from build123d import *

# Parameters (mm, degrees)
SKETCH1_R                  = 3.3782
BASE_FLANGE1_DEPTH         = 3.175
SKETCHED_START             = -12.7
SKETCHED_BEND1_DEPTH       = 25.4
SKETCHED_START_2           = -10.229596
SKETCHED_BEND1_2_DEPTH     = 6.8513959
SKETCHED_START_3           = 3.3782001
SKETCHED_BEND1_3_DEPTH     = 6.7817999
SKETCHED_BEND1_4_DEPTH     = 25.4
SKETCHED_START_4           = 9.775295033
SKETCHED_BEND1_5_OUTLINE_R = 3.3782
SKETCHED_BEND1_5_DEPTH     = 3.175


with BuildPart() as part:
    # Base-Flange1: sheet metal written as solids
    # Sketch1 → Base-Flange1 (new body)
    with BuildSketch(Plane.XY):
        with BuildLine():
            Line((-10.16, -25.4), (10.16, -25.4))
            ThreePointArc((10.16, -25.4), (11.956051224, -24.656051224), (12.7, -22.86))
            Line((12.7, -22.86), (12.7, 46.99))
            ThreePointArc((12.7, 46.99), (11.956051224, 48.786051224), (10.16, 49.53))
            Line((10.16, 49.53), (-10.16, 49.53))
            ThreePointArc((-10.16, 49.53), (-11.956051224, 48.786051224), (-12.7, 46.99))
            Line((-12.7, 46.99), (-12.7, -22.86))
            ThreePointArc((-12.7, -22.86), (-11.956051224, -24.656051224), (-10.16, -25.4))
        make_face()
        with Locations((0, 36.83)):
            Circle(SKETCH1_R, mode=Mode.SUBTRACT)
        with Locations((0, -12.7)):
            Circle(SKETCH1_R, mode=Mode.SUBTRACT)
    extrude(amount=-BASE_FLANGE1_DEPTH)

    # Sketched Bend1: read off the stored shape, not the designer's step
    # Sketched Bend1 outline → Sketched Bend1 (cut)
    with BuildSketch(Plane.YZ.offset(SKETCHED_START)):
        with BuildLine():
            Line((49.53, 0), (14.953712647, 0))
            Line((14.953712647, 0), (14.325844229, -1.0875))
            ThreePointArc((14.325844229, -1.0875), (12.797688168, -2.615656061), (10.710188168, -3.175))
            Line((10.710188168, -3.175), (49.53, -3.175))
            Line((49.53, -3.175), (49.53, 0))
        make_face()
    extrude(amount=SKETCHED_BEND1_DEPTH, mode=Mode.SUBTRACT)

    # Sketched Bend1 2 outline → Sketched Bend1 2 (add)
    with BuildSketch(Plane.YZ.offset(SKETCHED_START_2)):
        with BuildLine():
            Line((29.631307656, 31.772340289), (11.576213572, 0.5))
            ThreePointArc((11.576213572, 0.5), (11.210188168, 0.133974596), (10.710188168, 0))
            Line((10.710188168, 0), (14.953712647, 0))
            Line((14.953712647, 0), (32.380938313, 30.184840289))
            Line((32.380938313, 30.184840289), (29.631307656, 31.772340289))
        make_face()
    extrude(amount=SKETCHED_BEND1_2_DEPTH)

    # Sketched Bend1 3 outline → Sketched Bend1 3 (add)
    with BuildSketch(Plane.YZ.offset(SKETCHED_START_3)):
        with BuildLine():
            Line((29.631307656, 31.772340289), (11.576213572, 0.5))
            ThreePointArc((11.576213572, 0.5), (11.210188168, 0.133974596), (10.710188168, 0))
            Line((10.710188168, 0), (14.953712647, 0))
            Line((14.953712647, 0), (32.380938313, 30.184840289))
            Line((32.380938313, 30.184840289), (29.631307656, 31.772340289))
        make_face()
    extrude(amount=SKETCHED_BEND1_3_DEPTH)

    # Sketched Bend1 4 outline → Sketched Bend1 4 (add)
    with BuildSketch(Plane.YZ.offset(SKETCHED_START)):
        with BuildLine():
            Line((29.631307656, 31.772340289), (11.576213572, 0.5))
            ThreePointArc((11.576213572, 0.5), (11.210188168, 0.133974596), (10.710188168, 0))
            Line((10.710188168, 0), (14.953712647, 0))
            Line((14.953712647, 0), (32.380938313, 30.184840289))
            Line((32.380938313, 30.184840289), (29.631307656, 31.772340289))
        make_face()
    extrude(amount=SKETCHED_BEND1_4_DEPTH)

    # Sketched Bend1 5 outline → Sketched Bend1 5 (cut)
    with BuildSketch(Plane(origin=(0, 0, 0), x_dir=(1, 0, 0), z_dir=(0, 0.8660254037844399, -0.49999999999999795)).offset(SKETCHED_START_4)):
        with BuildLine():
            Line((-12.7, -42.331307656), (-10.16, -42.331307656))
            ThreePointArc((-10.16, -42.331307656), (-11.956051224, -41.58735888), (-12.7, -39.791307656))
            Line((-12.7, -39.791307656), (-12.7, -42.331307656))
        make_face()
        with BuildLine():
            ThreePointArc((12.7, -39.791307656), (11.956051224, -41.58735888), (10.16, -42.331307656))
            Line((10.16, -42.331307656), (12.7, -42.331307656))
            Line((12.7, -42.331307656), (12.7, -39.791307656))
        make_face()
        with Locations((0, -29.631307656)):
            Circle(SKETCHED_BEND1_5_OUTLINE_R)
    extrude(amount=SKETCHED_BEND1_5_DEPTH, mode=Mode.SUBTRACT)


solid = part.part
Design review of the part built by this model. Coordinates are the model's own, in mm. Give positions to 0.01 mm unless a question says otherwise; leave off trailing zeros. Order: outer loops, then holes, each group sorted by start corner. A loop starts at its lowest first (then second) coordinate and runs counter-clockwise, first axis right, second up. Notation, with made-up numbers: (80, -12.75) - (98, -12.75) arc R23 ccw to (98, 25.25) - close; hole circle Ø7 at (13.5, 25). An arc over 180 degrees is marked (long way). Write item = value, one per line. Start each with the question number.
Q1. Mouldability with a two-part tool opening along X and no side actions: class faces 1 (the face through (1.816, 23.213, 17.524)), 2 (the face through (12, 30.6, 30.3)), 3 (the face through (-0.73, -16, -1.57)), 4 (the face through (0, -7, 0)) as released by +X, released by -X, zero draft, split by the parting line, or undercut.
Q2. We need section D-D on y = 2. State the section outline as (x, z) points (3 decimals), plus the area to 3 significant figures.
Q3. Clearance check with flat-ended pins moving along their axes: pin 1 Ø5 at (x, y) = (-0.5, 25) entering from -Z; pin 2 Ø12 at (x, y) = (-8, 22.5) entering from +Z; pin 3 Ø8 at (x, z) = (-1, 22) entering from +Y. State where each tip first meets the part, or that it passes through.
Q4. To check wall thickness, follow L1, parallel to Z at x = 1.5, y = 1 (3 decimals); L2, parallel to Y at x = 0, z = -0.9; L3, parallel to Y at x = 0, z = -1.15. State the ranges of each line that lie inside material, in increasing order. Write a range as from..to.
Q5. We need section B-B on x = -2.25. State how many separate pieces and enclosed holes the cut face has, plus the area to 3 significant figures.
Q6. We need section A-A on y = -12.7. State the section outline as (x, z) points (3 decimals).
Working result:
q1.face_1 = undercut
q1.face_2 = released by +X
q1.face_3 = undercut
q1.face_4 = zero draft
q2.outline = (-12.7, -3.175) - (12.7, -3.175) - (12.7, 0) - (-12.7, 0) - close
q2.area = 80.6 mm²
q3.pin_1 = 13.07
q3.pin_2 = 29.81
q3.pin_3 = 29.96
q4.L1 = -3.175..0
q4.L2 = -25.4..-16.08, -9.32..14.43
q4.L3 = -25.4..-16.08, -9.32..14.29
q5.separate_pieces = 3
q5.enclosed_holes = 0
q5.area = 206 mm²
q6.outline = (-12.7, -3.175) - (-3.378, -3.175) - (-3.378, 0) - (-12.7, 0) - close; (3.378, -3.175) - (12.7, -3.175) - (12.7, 0) - (3.378, 0) - close
